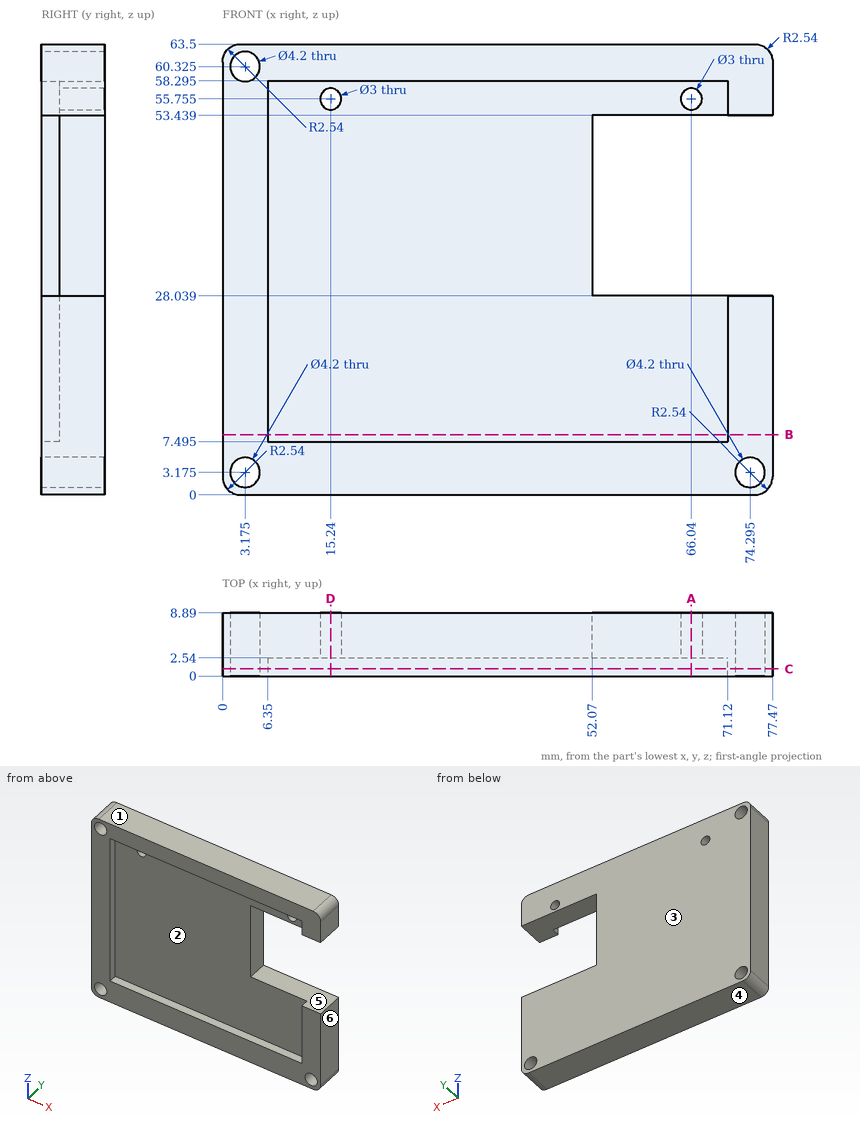
Can you work these out from the drawing? Everything is in mm from the part's minimum corner. A direction names the side the tool comes from. Give positions to 0.01 mm unless a question says otherwise; leave off trailing zeros. Order: outer loops, then holes, each group sorted by start corner. A loop starts at its lowest first (then second) coordinate and runs counter-clockwise, first axis right, second up.
Item 1: If we section it at C-C, the plane y = 1: Count the separate pieces of the cut face and the enclosed holes in it, plus the area to 3 significant figures.
Item 2: If we section it at D-D, the plane x = 15.24: Write out the boundary of the cut face in (y, z) (1 decimal).
Item 3: I'm going to push a flat-ended pin straight in: pin 1 (2 mm diameter, centred on y = 1.5, z = 44, fed in from +X). Where does the tip first touch, or does it pass through?
Item 4: I need wall thicknesses on line 1 (X direction, y = 2, z = 26); line 2 (Z direction, x = 5, y = 5) (1 decimal); line 3 (Z direction, x = 57, y = 4). Which ranges of each line are inside material? Lowest first, please.
Item 5: If we section it at A-A, the plane x = 66.04: Write out the boundary of the cut face in (y, z) (1 decimal).
Item 6: If we mould it in two halves opening along Z, with no side actions, what happens to the marked faces 1, 2, 3 and 4? For each: pulls with the +Z half, pulls with the -Z half, needs draft (parallel to the pull), parting line crosses it, or undercut.
Item 7: If we section it at B-B, the plane z = 8.5: Write out the boundary of the cut face in (x, y), plus the area to 3 significant figures.
Item 8: For the marked faces 5 and 6, which set-ups out of +Z, -Z, +X, -X, +Y, -Y let a thin tool reach every point of the face, with its end or its side?
Values:
1. separate pieces: 1
1. enclosed holes: 3
1. area: 1,420 mm2
2. outline: (0, 0) - (8.9, 0) - (8.9, 54.3) - (2.5, 54.3) - (2.5, 7.5) - (0, 7.5) - close; (0, 58.3) - (2.5, 58.3) - (2.5, 57.3) - (8.9, 57.3) - (8.9, 63.5) - (0, 63.5) - close
3. pin 1: stops at x = 6.35
4. line 1: x = 0 to 6.35, 71.12 to 77.47
4. line 2: z = 0 to 2.1, 4.2 to 59.3, 61.4 to 63.5
4. line 3: z = 0 to 28.04, 53.44 to 63.5
5. outline: (0, 0) - (8.9, 0) - (8.9, 28) - (2.5, 28) - (2.5, 7.5) - (0, 7.5) - close; (0, 58.3) - (2.5, 58.3) - (2.5, 57.3) - (8.9, 57.3) - (8.9, 63.5) - (0, 63.5) - close; (2.5, 53.4) - (8.9, 53.4) - (8.9, 54.3) - (2.5, 54.3) - close
6. face 1: pulls with the +Z half
6. face 2: undercut
6. face 3: needs draft
6. face 4: pulls with the -Z half
7. outline: (0, 0) - (6.35, 0) - (6.35, 2.54) - (71.12, 2.54) - (71.12, 0) - (77.47, 0) - (77.47, 8.89) - (0, 8.89) - close
7. area: 524 mm2
8. face 5: +X, +Y, -Y
8. face 6: +Z, -Z, +X, +Y, -Y
